```python
from build123d import *

# Parameters (mm, degrees)
F2_SIZE2 = 2.1435935394
F2_SIZE  = 8
F4_D     = 4.5
F4_DEPTH = 30
F4_TIP   = 1.3519363928


with BuildPart() as f1:
    # F0 (on Front) → F1 (revolve)
    with BuildSketch(Plane.XZ):
        Polygon((0, 50), (0, 0), (7.5, 0), (7.5, 32.2), (5.75, 32.2), (5.75, 40), (4.45, 40), (4.45, 50), align=None)
    revolve(axis=Axis((0, 0, 25), (0, 0, 1)))

    # F2
    f2_edges = [f1.edges().sort_by_distance(p)[0] for p in [
        (-4.45, 0, 50),
    ]]
    chamfer(f2_edges, length=F2_SIZE, length2=F2_SIZE2)

    # F4
    with Locations(Plane(origin=(0, 0, 0), x_dir=(1, 0, 0), z_dir=(0, 0, -1))):
        with Locations((0, 0)):
            Hole(F4_D / 2, depth=F4_DEPTH)
            with Locations((0, 0, -(F4_DEPTH + F4_TIP / 2))):  # 118° drill point
                Cone(0, F4_D / 2, F4_TIP, mode=Mode.SUBTRACT)


solid = f1.part
```
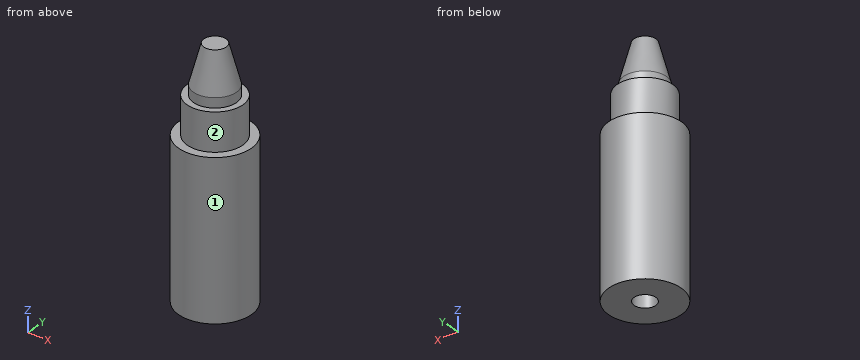
Build history of the part. All positions in model axes, mm. Face numbers are marked on the shaded views. A direction names the side the tool comes from. Round coordinates to 2 decimals unless told otherwise and drop trailing zeros. Write each loop counter-clockwise with the first axis right and the second up, starting at its lowest first coordinate (ties: lowest second). Pieces come first, ordered by that corner, then holes. Notation, with made-up numbers: (-12.75, 31) - (2.25, 31) arc R20 cw to (2.25, 35) - close; hole circle Ø7 at (-11, -12.75). An arc over 180 degrees is marked (long way). Answer as CSV lines item,"result".
Q1. Cut at A-A (x = 5). Write the cut outline in (y, z).
Report:
outline,"(-5.59, 0) - (5.59, 0) - (5.59, 32.2) - (2.84, 32.2) - (2.84, 40) - (-2.84, 40) - (-2.84, 32.2) - (-5.59, 32.2) - close"
Q2. Cut at B-B (z = 17). Write the cut outline in (x, y).
Report:
outline,"circle Ø15 at (0, 0); hole circle Ø4.5 at (0, 0)"
Q3. Tool access for the marked faces 1 and 2: list every direction of +Z, -Z, +X, -X, +Y, -Y with a clear straight run to the whole face (end or side of a thin tool).
Report:
face 1,"+Z, -Z"
face 2,"+Z"
Q4. Drop flat-ended pins along their axis: pin 1 (5 mm diameter, centred on y = 1, z = 35, fed in from -X); pin 2 (1.5 mm diameter, centred on x = 5, y = -4.5, fed in from +Z); pin 3 (3 mm diameter, centred on y = -3, z = 9.5, fed in from +X). Give the stop position or say it passes through.
Report:
pin 1,"stops at x = -5.75"
pin 2,"stops at z = 32.2"
pin 3,"stops at x = 7.35"
Q5. Drill centre lines: probe 1 along Y at (x, z) = (0, 13.25); probe 2 along Z at (x, y) = (2.75, -4.25); probe 3 along Z at (x, y) = (-6.75, 1.75). Where is each one in solid material? Low to high. Write a range as [from, to].
Report:
probe 1,"y = [-7.5, -2.25], [2.25, 7.5]"
probe 2,"z = [0, 40]"
probe 3,"z = [0, 32.2]"
